from build123d import *

# Parameters (mm, degrees)
ESQUISSE1_R                  = 160
BOSS_EXTRU_1_DEPTH           = 7.5
ESQUISSE2_R                  = 110.25
ENL_V_MAT_EXTRU_1_DEPTH      = 2
ESQUISSE3_R                  = 1.6
ENL_V_MAT_EXTRU_2_DEPTH      = 14
R_P_TITION_CIRCULAIRE1_COUNT = 3
ESQUISSE4_R                  = 1
ENL_V_MAT_EXTRU_3_DEPTH      = 14
ESQUISSE10_R                 = 5
ENL_V_MAT_EXTRU_6_DEPTH      = 11
ESQUISSE11_R                 = 160
ESQUISSE11_R_2               = 156
ENL_V_MAT_EXTRU_7_DEPTH      = 4
ESQUISSE8_R                  = 26.25
ENL_V_MAT_EXTRU_4_DEPTH      = 2
R_P_TITION_CIRCULAIRE2_COUNT = 9
ESQUISSE9_R                  = 26.25
ENL_V_MAT_EXTRU_5_DEPTH      = 2
R_P_TITION_CIRCULAIRE3_COUNT = 4


with BuildPart() as part:
    # Esquisse1 → Boss.-Extru.1 (new body, symmetric)
    with BuildSketch(Plane(origin=(0, 0, 0), x_dir=(1, 0, 0), z_dir=(0, 1, 0))):
        Circle(ESQUISSE1_R)
    extrude(amount=BOSS_EXTRU_1_DEPTH, both=True)

    # Esquisse2 → Enlèv. mat.-Extru.1 (cut)
    with BuildSketch(Plane.XZ.offset(7.5)):
        Circle(ESQUISSE2_R)
    extrude(amount=-ENL_V_MAT_EXTRU_1_DEPTH, mode=Mode.SUBTRACT)

    # Esquisse3 → Enlèv. mat.-Extru.2 (cut, through all)
    with BuildSketch(Plane(origin=(0, -5.5, 0), x_dir=(-1, 0, 0), z_dir=(0, -1, 0))):
        with Locations((0, -106.8)):
            Circle(ESQUISSE3_R)
    enl_v_mat_extru_2 = extrude(amount=-ENL_V_MAT_EXTRU_2_DEPTH, mode=Mode.SUBTRACT)

    # Répétition circulaire1: Enlèv. mat.-Extru.2 ×3 about axis
    r_p_tition_circulaire1_axis = Axis((0, 0, 0), (0, 1, 0))
    for i in range(1, R_P_TITION_CIRCULAIRE1_COUNT):
        add(enl_v_mat_extru_2.rotate(r_p_tition_circulaire1_axis, i * 360 / R_P_TITION_CIRCULAIRE1_COUNT), mode=Mode.SUBTRACT)

    # Esquisse4 → Enlèv. mat.-Extru.3 (cut, through all)
    with BuildSketch(Plane.XZ.offset(5.5)):
        Circle(ESQUISSE4_R)
    extrude(amount=-ENL_V_MAT_EXTRU_3_DEPTH, mode=Mode.SUBTRACT)

    # Esquisse10 → Enlèv. mat.-Extru.6 (cut)
    with BuildSketch(Plane(origin=(0, 7.5, 0), x_dir=(1, 0, 0), z_dir=(0, 1, 0))):
        Circle(ESQUISSE10_R)
    extrude(amount=-ENL_V_MAT_EXTRU_6_DEPTH, mode=Mode.SUBTRACT)

    # Esquisse11 → Enlèv. mat.-Extru.7 (cut)
    with BuildSketch(Plane(origin=(0, -7.5, 0), x_dir=(1, 0, 0), z_dir=(0, 1, 0))):
        Circle(ESQUISSE11_R)
        Circle(ESQUISSE11_R_2, mode=Mode.SUBTRACT)
    enl_v_mat_extru_7 = extrude(amount=ENL_V_MAT_EXTRU_7_DEPTH, mode=Mode.SUBTRACT)

    # Symétrie1: Enlèv. mat.-Extru.7 across plane
    add(enl_v_mat_extru_7.mirror(Plane.ZX), mode=Mode.SUBTRACT)

    # Esquisse8 → Enlèv. mat.-Extru.4 (cut)
    with BuildSketch(Plane(origin=(0, 7.5, 0), x_dir=(1, 0, 0), z_dir=(0, 1, 0))):
        with Locations((0, 115)):
            Circle(ESQUISSE8_R)
    enl_v_mat_extru_4 = extrude(amount=-ENL_V_MAT_EXTRU_4_DEPTH, mode=Mode.SUBTRACT)

    # Répétition circulaire2: Enlèv. mat.-Extru.4 ×9 about axis
    r_p_tition_circulaire2_axis = Axis((0, 0, 0), (0, 1, 0))
    for i in range(1, R_P_TITION_CIRCULAIRE2_COUNT):
        add(enl_v_mat_extru_4.rotate(r_p_tition_circulaire2_axis, i * 360 / R_P_TITION_CIRCULAIRE2_COUNT), mode=Mode.SUBTRACT)

    # Esquisse9 → Enlèv. mat.-Extru.5 (cut)
    with BuildSketch(Plane(origin=(0, 7.5, 0), x_dir=(1, 0, 0), z_dir=(0, 1, 0))):
        with Locations((0, 48)):
            Circle(ESQUISSE9_R)
    enl_v_mat_extru_5 = extrude(amount=-ENL_V_MAT_EXTRU_5_DEPTH, mode=Mode.SUBTRACT)

    # Répétition circulaire3: Enlèv. mat.-Extru.5 ×4 about axis
    r_p_tition_circulaire3_axis = Axis((0, 0, 0), (0, 1, 0))
    for i in range(1, R_P_TITION_CIRCULAIRE3_COUNT):
        add(enl_v_mat_extru_5.rotate(r_p_tition_circulaire3_axis, i * 360 / R_P_TITION_CIRCULAIRE3_COUNT), mode=Mode.SUBTRACT)


solid = part.part
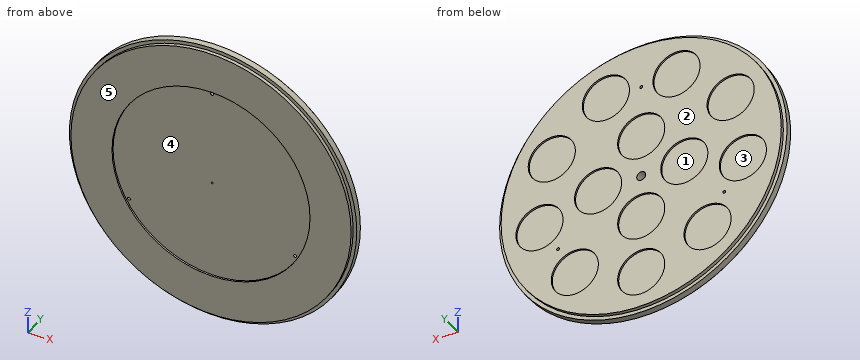
Input: part model. Units: mm. Frame: model coordinates. Face numbers are marked on the shaded views. A direction names the side the tool comes from. Give positions to 0.01 mm unless a question says otherwise; leave off trailing zeros. Write each loop counter-clockwise with the first axis right and the second up, starting at its lowest first coordinate (ties: lowest second). Pieces come first, ordered by that corner, then holes. Notation, with made-up numbers: M -15.5,-11 L 24.5,-11 A11 ccw 24.5,-5 Z; hole C -7.5,34 d1. An arc over 180 degrees is marked long. Use one line per item in the form item = value.
1. Cut plane C-C on y = 0.75. Return loops of the section in (x, z), and give its area (3 significant figures).
Outcome:
outline = C 0,0 d320; hole C -92.49,-53.4 d3.2; hole C 0,0 d10; hole C 0,106.8 d3.2; hole C 92.49,-53.4 d3.2
area = 80,300 mm²
2. Cut plane D-D on z = 57.5. Return loops of the section in (x, y).
Outcome:
outline = M -149.31,-3.5 L -145.02,-3.5 L -145.02,-7.5 L -94.07,-7.5 L -94.07,-5.5 L 94.07,-5.5 L 94.07,-7.5 L 145.02,-7.5 L 145.02,-3.5 L 149.31,-3.5 L 149.31,3.5 L 145.02,3.5 L 145.02,7.5 L 125.84,7.5 L 125.84,5.5 L 73.34,5.5 L 73.34,7.5 L 24.47,7.5 L 24.47,5.5 L -24.47,5.5 L -24.47,7.5 L -73.34,7.5 L -73.34,5.5 L -125.84,5.5 L -125.84,7.5 L -145.02,7.5 L -145.02,3.5 L -149.31,3.5 Z
3. Cut plane B-B on z = 92. Return loops of the section in (x, y).
Outcome:
outline = M -130.9,-3.5 L -125.98,-3.5 L -125.98,-7.5 L -60.75,-7.5 L -60.75,-5.5 L 60.75,-5.5 L 60.75,-7.5 L 125.98,-7.5 L 125.98,-3.5 L 130.9,-3.5 L 130.9,3.5 L 125.98,3.5 L 125.98,7.5 L 60.09,7.5 L 60.09,5.5 L 18.57,5.5 L 18.57,7.5 L -18.57,7.5 L -18.57,5.5 L -60.09,5.5 L -60.09,7.5 L -125.98,7.5 L -125.98,3.5 L -130.9,3.5 Z
4. Reachability of the marked faces 3, 4 and 5 from +Z, -Z, +X, -X, +Y, -Y: full face, straight path, thin tool, end or side. Return the list, or none.
Outcome:
face_3 = +Y
face_4 = -Y
face_5 = +Z, -Z, +X, -X, -Y
5. First-contact query: P1, Ø4, axis at x = 83.5, y = -0.5, coming from the -Z side; P2, Ø2, axis at y = 2, z = -46, coming from the +X side; P3, Ø3, axis at y = -4, z = -7.5, coming from the +X side. Flat tips, straight axial feed; report the tip coordinate or a pass-through.
Outcome:
P1 = -137.69
P2 = 153.54
P3 = 159.88
6. Cut plane A-A on x = -83. Return loops of the section in (y, z), and give its area (3 significant figures).
Outcome:
outline = M -7.5,-132.09 L -3.5,-132.09 L -3.5,-136.79 L 3.5,-136.79 L 3.5,-132.09 L 7.5,-132.09 L 7.5,-112.72 L 5.5,-112.72 L 5.5,-63.47 L 7.5,-63.47 L 7.5,37.16 L 5.5,37.16 L 5.5,77.84 L 7.5,77.84 L 7.5,132.09 L 3.5,132.09 L 3.5,136.79 L -3.5,136.79 L -3.5,132.09 L -7.5,132.09 L -7.5,72.57 L -5.5,72.57 L -5.5,-72.57 L -7.5,-72.57 Z
area = 3,560 mm²
7. Ray query, L1, parallel to Z at x = 0, y = 6.9; L2, parallel to X at y = 3, z = 0; L3, parallel to Y at x = 43, z = 62.5. Return the intervals inside material, ascending.
Outcome:
L1 = -156 to -141.25, -88.75 to -74.25, -21.75 to -5, 5 to 21.75, 74.25 to 105.2, 108.4 to 156
L2 = -160 to -5, 5 to 160
L3 = -5.5 to 7.5
8. Mould query, pull axis X, two halves, no side actions, for the marked faces 1 and 2. Classes: released by +X, released by -X, zero draft, split by the parting line, or undercut.
Outcome:
face_1 = undercut
face_2 = zero draft
